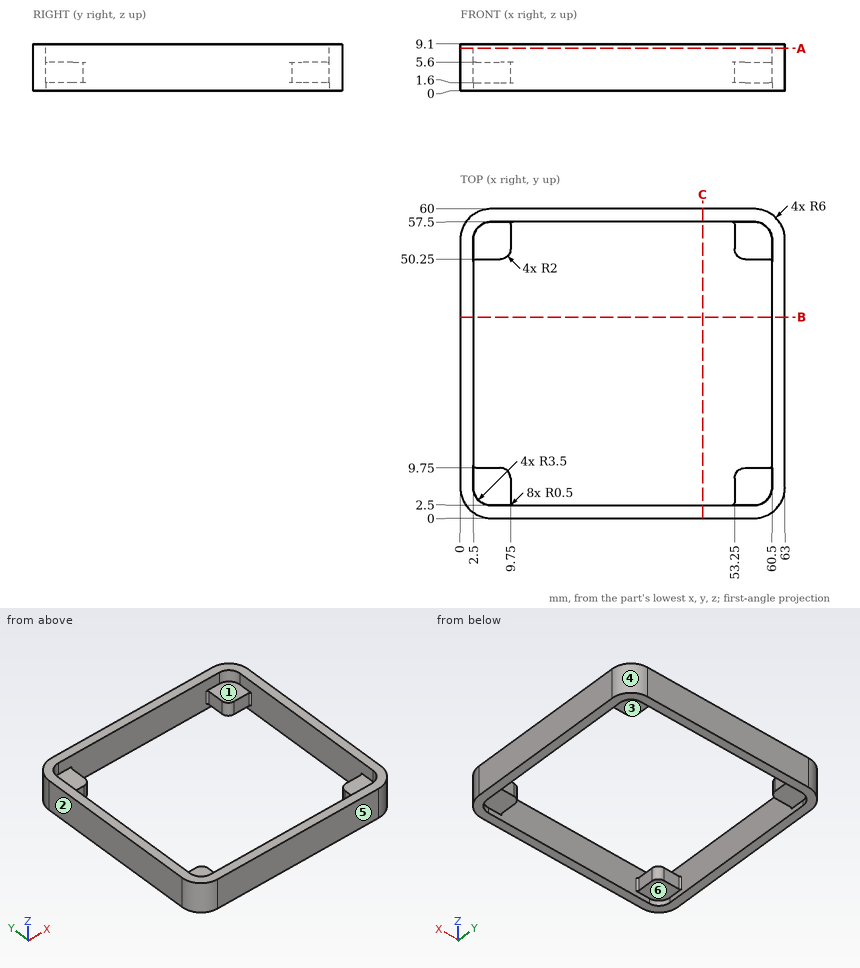
Answer from the drawing. Dimensions are ordinates in mm from the lowest x, y and z of the part. A direction names the side the tool comes from. Give positions to 0.01 mm unless a question says otherwise; leave off trailing zeros. Order: outer loops, then holes, each group sorted by start corner. A loop starts at its lowest first (then second) coordinate and runs counter-clockwise, first axis right, second up. Notation, with made-up numbers: (13.5, 79.5) - (37.5, 79.5) arc R25 cw to (37.5, 97.5) - close; hole circle Ø4 at (-4.5, 80.5). An arc over 180 degrees is marked (long way). One line per item, written item: value. Start each with the question number.
1. Section B-B, the plane y = 39 is taken. Write down the section's boundary in (x, z), then the cut area to 3 significant figures.
2. Consider line 1 (Y direction, x = 23.5, z = 8.5); line 2 (X direction, y = 52.5, z = 8.25); line 3 (X direction, y = 56, z = 4). Determine where each line is inside the solid, lowest interval first.
3. For a pull along X with two mould halves and no side action, classify the marked faces 4, 5 and 6 as released by +X, released by -X, zero draft, split by the parting line, or undercut.
4. Which of the six approach directions +Z, -Z, +X, -X, +Y, -Y give full straight-line access (tool end or side, diameter ignored) to the marked faces 1, 2 and 3?
5. Section C-C, the plane x = 47 is taken. Write down the section's boundary in (y, z).
6. Section A-A, the plane z = 8.25 is taken. Write down the section's boundary in (x, y), then the cut area to 3 significant figures.
7. Each of these flat-tipped pins is pushed along its axis until it touches: pin 1 Ø12 at (x, y) = (31, 53) entering from -Z; pin 2 Ø6 at (x, y) = (7.5, 52) entering from -Z; pin 3 Ø1.2 at (x, z) = (4.5, 2.5) entering from +Y; pin 4 Ø2 at (y, z) = (4.5, 3) entering from +X. Where does it stop, or does it pass through?
Filled sheet:
1. outline: (0, 0) - (2.5, 0) - (2.5, 9.1) - (0, 9.1) - close; (60.5, 0) - (63, 0) - (63, 9.1) - (60.5, 9.1) - close
1. area: 45.5 mm²
2. line 1: 0 to 2.5, 57.5 to 60
2. line 2: 0 to 2.5, 60.5 to 63
2. line 3: 0.34 to 9.75, 53.25 to 62.66
3. face 4: released by +X
3. face 5: zero draft
3. face 6: undercut
4. face 1: +Z
4. face 2: +Z, -Z, -X, +Y, -Y
4. face 3: -Z
5. outline: (0, 0) - (2.5, 0) - (2.5, 9.1) - (0, 9.1) - close; (57.5, 0) - (60, 0) - (60, 9.1) - (57.5, 9.1) - close
6. outline: (0, 6) arc R6 ccw to (6, 0) - (57, 0) arc R6 ccw to (63, 6) - (63, 54) arc R6 ccw to (57, 60) - (6, 60) arc R6 ccw to (0, 54) - close; hole (2.5, 6) arc R3.5 ccw to (6, 2.5) - (57, 2.5) arc R3.5 ccw to (60.5, 6) - (60.5, 54) arc R3.5 ccw to (57, 57.5) - (6, 57.5) arc R3.5 ccw to (2.5, 54) - close
6. area: 570 mm²
7. pin 1: z = 0
7. pin 2: z = 1.6
7. pin 3: y = 59.93
7. pin 4: x = 62.98
